Check sheet for the modelled part. Datum: model origin and axes. Units: mm. A direction names the side the tool comes from. Give positions to 0.01 mm unless a question says otherwise; leave off trailing zeros. Write each loop counter-clockwise with the first axis right and the second up, starting at its lowest first coordinate (ties: lowest second). Pieces come first, ordered by that corner, then holes. Notation, with made-up numbers: (87.5, 40) -> (109.5, 40) arc R17 cw to (109.5, 63) -> close; hole circle Ø4 at (-12, -8). An arc over 180 degrees is marked (long way). Return JSON: item names as keys, results as strings.
from build123d import *

# Parameters (mm, degrees)
SKETCH1_W               = 30
SKETCH1_H               = 30
BOSS_EXTRUDE1_DEPTH     = 10
SKETCH2_W               = 31
SKETCH2_H               = 31
SKETCH2_W_2             = 15
SKETCH2_H_2             = 15
CUT_EXTRUDE1_DEPTH      = 8
FILLET1_R               = 1
CUT_EXTRUDE2_DEPTH      = 28.820855486
CUT_EXTRUDE2_DEPTH_BACK = 28.820855486
SKETCH3_R               = 2.5


with BuildPart() as part:
    # Sketch1 → Boss-Extrude1 (new, symmetric)
    with BuildSketch(Plane(origin=(0, 0, 0), x_dir=(1, 0, 0), z_dir=(0, 1, 0))):
        Rectangle(SKETCH1_W, SKETCH1_H)
    extrude(amount=BOSS_EXTRUDE1_DEPTH, both=True)

    # Sketch2 → Cut-Extrude1 (cut, symmetric)
    # profile 1 of 3: a face of its own
    with BuildSketch(Plane(origin=(0, 0, 0), x_dir=(1, 0, 0), z_dir=(0, 1, 0))):
        with Locations((-7.5, 7.5)):
            Rectangle(SKETCH2_W, SKETCH2_H)
        with Locations((-7.5, 7.5)):
            Rectangle(SKETCH2_W_2, SKETCH2_H_2, mode=Mode.SUBTRACT)
    # profile 2 of 3: a face of its own
    with BuildSketch(Plane(origin=(0, 0, 0), x_dir=(1, 0, 0), z_dir=(0, 1, 0))):
        with Locations((-7.5, 7.5)):
            Rectangle(SKETCH2_W, SKETCH2_H)
        with Locations((-7.5, 7.5)):
            Rectangle(SKETCH2_W_2, SKETCH2_H_2, mode=Mode.SUBTRACT)
    # profile 3 of 3: a face of its own
    with BuildSketch(Plane(origin=(0, 0, 0), x_dir=(1, 0, 0), z_dir=(0, 1, 0))):
        with Locations((-7.5, 7.5)):
            Rectangle(SKETCH2_W_2, SKETCH2_H_2)
    extrude(amount=CUT_EXTRUDE1_DEPTH, both=True, mode=Mode.SUBTRACT)

    # Fillet1
    fillet1_edges = [part.edges().sort_by_distance(p)[0] for p in [
        (8, 0, 8),
    ]]
    fillet(fillet1_edges, radius=FILLET1_R)

    # Sketch3 → Cut-Extrude2 (cut, two sides: drawn at the far end of the back side and taken through both)
    with BuildSketch(Plane(origin=(0, -8, 0), x_dir=(1, 0, 0), z_dir=(0, 1, 0)).offset(-CUT_EXTRUDE2_DEPTH_BACK)):
        with Locations(Location((-2, 1, 0), (0, 0, 270))):
            Circle(SKETCH3_R)
    extrude(amount=CUT_EXTRUDE2_DEPTH + CUT_EXTRUDE2_DEPTH_BACK, mode=Mode.SUBTRACT)


solid = part.part
(1) Cross-section at D-D on z = 6.5. Enter the section's corners in (x, y), then the cut area to 3 significant figures.
Reply:
{"outline": "(-15, -10) -> (15, -10) -> (15, 10) -> (-15, 10) -> (-15, 8) -> (8, 8) -> (8, -8) -> (-15, -8) -> close", "area": "232 mm^2"}
(2) Depth check by flat-ended pin: pin 1 Ø5 at (y, z) = (2, -2) entering from -X; pin 2 Ø5 at (x, y) = (-6.5, 3.5) entering from -Z. Enter the tip coordinate at first touch or a pass-through.
Reply:
{"pin 1": "x = 8", "pin 2": "z = 8"}
(3) Set-up check for faces 1 (the flat face through (15, 0, 0)), 2 (the flat face through (-4, 0, 8)): record each of +Z, -Z, +X, -X, +Y, -Y from which the full face is reachable in a straight line by a thin tool's end or side.
Reply:
{"face 1": "+Z, -Z, +X, +Y, -Y", "face 2": "-Z, -X"}
(4) Cross-section at B-B on z = -1. Enter the section's corners in (x, y).
Reply:
{"outline": "(-15, -10) -> (-4.5, -10) -> (-4.5, -8) -> (-15, -8) -> close; (-15, 8) -> (-4.5, 8) -> (-4.5, 10) -> (-15, 10) -> close; (0.5, -10) -> (15, -10) -> (15, 10) -> (0.5, 10) -> (0.5, 8) -> (8, 8) -> (8, -8) -> (0.5, -8) -> close"}
(5) Cross-section at A-A on x = -2. Enter the section's corners in (y, z), then the cut area to 3 significant figures.
Reply:
{"outline": "(-10, -15) -> (-8, -15) -> (-8, -3.5) -> (-10, -3.5) -> close; (-10, 1.5) -> (-8, 1.5) -> (-8, 8) -> (8, 8) -> (8, 1.5) -> (10, 1.5) -> (10, 15) -> (-10, 15) -> close; (8, -15) -> (10, -15) -> (10, -3.5) -> (8, -3.5) -> close", "area": "212 mm^2"}
(6) Cross-section at C-C on y = -5.5. Enter the section's corners in (x, z), then the cut area to 3 significant figures.
Reply:
{"outline": "(-15, 8) -> (7, 8) arc R1 cw to (8, 7) -> (8, -15) -> (15, -15) -> (15, 15) -> (-15, 15) -> close", "area": "371 mm^2"}
(7) Thickness scan on L1, parallel to Y at x = 3, z = 4; L2, parallel to Z at x = -2, y = 9.1; L3, parallel to X at y = 9.2, z = -1. Record the ranges inside material, lowest first.
Reply:
{"L1": "-10 to -8, 8 to 10", "L2": "-15 to -3.5, 1.5 to 15", "L3": "-15 to -4.5, 0.5 to 15"}
(8) Release check for a two-part mould opening along Y. For faces 3 (the cylindrical face through (-4.22, 8.99, 0.15)), 4 (the cylindrical face through (7.699, 0.112, 7.715)), 5 (the flat face through (3, -10, 0)) record: pulls with the +Y half, pulls with the -Y half, needs draft (parallel to the pull), parting line crosses it, or undercut.
Reply:
{"face 3": "needs draft", "face 4": "undercut", "face 5": "pulls with the -Y half"}
